from build123d import *

# Parameters (mm, degrees)
MODEL_R             = 2.5
BOSS_EXTRUDE1_DEPTH = 240


with BuildPart() as part:
    # Model → Boss-Extrude1 (new body)
    with BuildSketch(Plane.XY):
        with BuildLine():
            Line((3.9, -0.3), (3.9, -2.310912704))
            ThreePointArc((3.9, -2.310912704), (4.052240935, -3.076279568), (4.485786438, -3.725126266))
            Line((4.485786438, -3.725126266), (6.560660172, -5.8))
            Line((6.560660172, -5.8), (7.9, -5.8))
            ThreePointArc((7.9, -5.8), (8.112132034, -5.712132034), (8.2, -5.5))
            Line((8.2, -5.5), (8.2, -3.7))
            ThreePointArc((8.2, -3.7), (8.287867966, -3.487867966), (8.5, -3.4))
            Line((8.5, -3.4), (9.2, -3.4))
            ThreePointArc((9.2, -3.4), (9.412132034, -3.487867966), (9.5, -3.7))
            Line((9.5, -3.7), (9.5, -3.6))
            Line((9.5, -3.6), (9.7, -3.6))
            ThreePointArc((9.7, -3.6), (9.912132034, -3.687867966), (10, -3.9))
            Line((10, -3.9), (10, -8.5))
            ThreePointArc((10, -8.5), (9.560660172, -9.560660172), (8.5, -10))
            Line((8.5, -10), (4.15825757, -10))
            ThreePointArc((4.15825757, -10), (3.907259562, -9.864316767), (3.883303028, -9.58))
            ThreePointArc((3.883303028, -9.58), (3.867332005, -9.390455488), (3.7, -9.3))
            ThreePointArc((3.7, -9.3), (3.487867966, -9.212132034), (3.4, -9))
            Line((3.4, -9), (3.4, -8.8))
            ThreePointArc((3.4, -8.8), (3.487867966, -8.587867966), (3.7, -8.5))
            Line((3.7, -8.5), (5.2, -8.5))
            ThreePointArc((5.2, -8.5), (5.412132034, -8.412132034), (5.5, -8.2))
            Line((5.5, -8.2), (5.5, -6.98492424))
            ThreePointArc((5.5, -6.98492424), (5.47716386, -6.870119211), (5.412132034, -6.772792206))
            Line((5.412132034, -6.772792206), (3.425126266, -4.785786438))
            ThreePointArc((3.425126266, -4.785786438), (2.776279568, -4.352240935), (2.010912703, -4.2))
            Line((2.010912703, -4.2), (0, -4.2))
            Line((0, -4.2), (-2.010912703, -4.2))
            ThreePointArc((-2.010912703, -4.2), (-2.776279568, -4.352240935), (-3.425126266, -4.785786438))
            Line((-3.425126266, -4.785786438), (-5.412132034, -6.772792206))
            ThreePointArc((-5.412132034, -6.772792206), (-5.47716386, -6.870119211), (-5.5, -6.984924241))
            Line((-5.5, -6.984924241), (-5.5, -8.2))
            ThreePointArc((-5.5, -8.2), (-5.412132034, -8.412132034), (-5.2, -8.5))
            Line((-5.2, -8.5), (-3.4, -8.5))
            ThreePointArc((-3.4, -8.5), (-3.187867966, -8.587867966), (-3.1, -8.8))
            Line((-3.1, -8.8), (-3.1, -9.2))
            ThreePointArc((-3.1, -9.2), (-3.187867966, -9.412132034), (-3.4, -9.5))
            ThreePointArc((-3.4, -9.5), (-3.541421356, -9.558578644), (-3.6, -9.7))
            ThreePointArc((-3.6, -9.7), (-3.687867966, -9.912132034), (-3.9, -10))
            Line((-3.9, -10), (-8.5, -10))
            ThreePointArc((-8.5, -10), (-9.560660172, -9.560660172), (-10, -8.5))
            Line((-10, -8.5), (-10, -3.9))
            ThreePointArc((-10, -3.9), (-9.912132034, -3.687867966), (-9.7, -3.6))
            Line((-9.7, -3.6), (-9.5, -3.6))
            Line((-9.5, -3.6), (-9.5, -3.7))
            ThreePointArc((-9.5, -3.7), (-9.412132034, -3.487867966), (-9.2, -3.4))
            Line((-9.2, -3.4), (-8.5, -3.4))
            ThreePointArc((-8.5, -3.4), (-8.287867966, -3.487867966), (-8.2, -3.7))
            Line((-8.2, -3.7), (-8.2, -5.5))
            ThreePointArc((-8.2, -5.5), (-8.112132034, -5.712132034), (-7.9, -5.8))
            Line((-7.9, -5.8), (-6.68492424, -5.8))
            ThreePointArc((-6.68492424, -5.8), (-6.570119211, -5.77716386), (-6.472792206, -5.712132034))
            Line((-6.472792206, -5.712132034), (-4.485786438, -3.725126266))
            ThreePointArc((-4.485786438, -3.725126266), (-4.052240935, -3.076279568), (-3.9, -2.310912704))
            Line((-3.9, -2.310912704), (-3.9, -0.3))
            Line((-3.9, -0.3), (-3.9, 1.710912703))
            ThreePointArc((-3.9, 1.710912703), (-4.052240935, 2.476279568), (-4.485786438, 3.125126266))
            Line((-4.485786438, 3.125126266), (-6.472792206, 5.112132034))
            ThreePointArc((-6.472792206, 5.112132034), (-6.570119211, 5.17716386), (-6.68492424, 5.2))
            Line((-6.68492424, 5.2), (-7.9, 5.2))
            ThreePointArc((-7.9, 5.2), (-8.112132034, 5.112132034), (-8.2, 4.9))
            Line((-8.2, 4.9), (-8.2, 3.4))
            ThreePointArc((-8.2, 3.4), (-8.287867966, 3.187867966), (-8.5, 3.1))
            Line((-8.5, 3.1), (-9.2, 3.1))
            ThreePointArc((-9.2, 3.1), (-9.412132034, 3.187867966), (-9.5, 3.4))
            Line((-9.5, 3.4), (-9.5, 3.6))
            Line((-9.5, 3.6), (-9.7, 3.6))
            ThreePointArc((-9.7, 3.6), (-9.912132034, 3.687867966), (-10, 3.9))
            Line((-10, 3.9), (-10, 8.5))
            ThreePointArc((-10, 8.5), (-9.560660172, 9.560660172), (-8.5, 10))
            Line((-8.5, 10), (-3.9, 10))
            ThreePointArc((-3.9, 10), (-3.687867966, 9.912132034), (-3.6, 9.7))
            Line((-3.6, 9.7), (-3.6, 9.5))
            Line((-3.6, 9.5), (-3.4, 9.5))
            ThreePointArc((-3.4, 9.5), (-3.187867966, 9.412132034), (-3.1, 9.2))
            Line((-3.1, 9.2), (-3.1, 8.7))
            ThreePointArc((-3.1, 8.7), (-3.187867966, 8.487867965), (-3.4, 8.4))
            Line((-3.4, 8.4), (-5.2, 8.4))
            ThreePointArc((-5.2, 8.4), (-5.412132034, 8.312132034), (-5.5, 8.1))
            Line((-5.5, 8.1), (-5.5, 6.38492424))
            ThreePointArc((-5.5, 6.38492424), (-5.47716386, 6.270119211), (-5.412132034, 6.172792206))
            Line((-5.412132034, 6.172792206), (-3.425126266, 4.185786438))
            ThreePointArc((-3.425126266, 4.185786438), (-2.776279568, 3.752240935), (-2.010912703, 3.6))
            Line((-2.010912703, 3.6), (0, 3.6))
            Line((0, 3.6), (2.010912703, 3.6))
            ThreePointArc((2.010912703, 3.6), (2.776279568, 3.752240935), (3.425126266, 4.185786438))
            Line((3.425126266, 4.185786438), (5.412132034, 6.172792206))
            ThreePointArc((5.412132034, 6.172792206), (5.47716386, 6.270119211), (5.5, 6.38492424))
            Line((5.5, 6.38492424), (5.5, 8.1))
            ThreePointArc((5.5, 8.1), (5.412132034, 8.312132034), (5.2, 8.4))
            Line((5.2, 8.4), (3.7, 8.4))
            ThreePointArc((3.7, 8.4), (3.487867966, 8.487867965), (3.4, 8.7))
            Line((3.4, 8.7), (3.4, 9.2))
            ThreePointArc((3.4, 9.2), (3.487867966, 9.412132034), (3.7, 9.5))
            Line((3.7, 9.5), (3.6, 9.5))
            Line((3.6, 9.5), (3.6, 9.7))
            ThreePointArc((3.6, 9.7), (3.687867966, 9.912132034), (3.9, 10))
            Line((3.9, 10), (8.5, 10))
            ThreePointArc((8.5, 10), (9.560660172, 9.560660172), (10, 8.5))
            Line((10, 8.5), (10, 3.9))
            ThreePointArc((10, 3.9), (9.912132034, 3.687867966), (9.7, 3.6))
            Line((9.7, 3.6), (9.5, 3.6))
            Line((9.5, 3.6), (9.5, 3.4))
            ThreePointArc((9.5, 3.4), (9.412132034, 3.187867966), (9.2, 3.1))
            Line((9.2, 3.1), (8.5, 3.1))
            ThreePointArc((8.5, 3.1), (8.287867966, 3.187867966), (8.2, 3.4))
            Line((8.2, 3.4), (8.2, 4.9))
            ThreePointArc((8.2, 4.9), (8.112132034, 5.112132034), (7.9, 5.2))
            Line((7.9, 5.2), (6.684924241, 5.2))
            ThreePointArc((6.684924241, 5.2), (6.570119211, 5.17716386), (6.472792206, 5.112132034))
            Line((6.472792206, 5.112132034), (4.485786438, 3.125126266))
            ThreePointArc((4.485786438, 3.125126266), (4.052240935, 2.476279568), (3.9, 1.710912703))
            Line((3.9, 1.710912703), (3.9, -0.3))
        make_face()
        with Locations((0, -0.3)):
            Circle(MODEL_R, mode=Mode.SUBTRACT)
    extrude(amount=BOSS_EXTRUDE1_DEPTH)


solid = part.part
Verification items for the finished model (mm, model axes). A direction names the side the tool comes from. Coordinates: 2 decimals unless noted, no trailing zeros. Order: outer loops, then holes, each group sorted by start corner. A loop starts at its lowest first (then second) coordinate and runs counter-clockwise, first axis right, second up. Notation, with made-up numbers: (51, -14) -> (110, -14) arc R17 cw to (110, 18) -> close; hole circle Ø7 at (-12, -13.75). An arc over 180 degrees is marked (long way). Put each result on its own line as item: value. Start each with the question number.
1. Cross-section at B-B, the plane x = 0. Record the boundary of the cut face in (y, z), then the cut area to 3 significant figures.
2. Access from +Z, -Z, +X, -X, +Y, -Y to the whole of each face (thin tool, end or side, straight path). Record for faces 1 (the flat face through (3.9, 0, 118)), 2 (the flat face through (0, 3.6, 118)), 3 (the flat face through (0, -4.2, 118)).
3. Go/stop test with flat-tipped pins: pin 1 Ø3 at (y, z) = (0, 167.5) entering from +X; pin 2 Ø4.5 at (x, z) = (-1, 76.5) entering from -Y; pin 3 Ø4 at (x, y) = (-4, 0.5) entering from +Z; pin 4 Ø5 at (x, z) = (-0.5, 134.5) entering from -Y. Record where each tip stops, or that it passes through.
4. Material ranges on L1, parallel to Y at x = 0, z = 144.5; L2, parallel to Y at x = 6.75, z = 166; L3, parallel to X at y = 6, z = 70.5, recorded low to high. Write a range as [from, to].
5. Cross-section at A-A, the plane y = -0.3. Record the boundary of the cut face in (x, z), then the cut area to 3 significant figures.
Computed:
1. outline: (-4.2, 0) -> (-2.8, 0) -> (-2.8, 240) -> (-4.2, 240) -> close; (2.2, 0) -> (3.6, 0) -> (3.6, 240) -> (2.2, 240) -> close
1. area: 672 mm2
2. face 1: +Z, -Z, +X
2. face 2: +Z, -Z, +Y
2. face 3: +Z, -Z, -Y
3. pin 1: x = 3.9
3. pin 2: y = -9.46
3. pin 3: z = 240
3. pin 4: y = -4.46
4. L1: [-4.2, -2.8], [2.2, 3.6]
4. L2: [-10, -5.8], [5.2, 10]
4. L3: [-10, -5.24], [5.24, 10]
5. outline: (-3.9, 0) -> (-2.5, 0) -> (-2.5, 240) -> (-3.9, 240) -> close; (2.5, 0) -> (3.9, 0) -> (3.9, 240) -> (2.5, 240) -> close
5. area: 672 mm2
